Input: dimensioned drawing with shaded views. Units: mm. Origin: part minimum x, y, z. A direction names the side the tool comes from. Give positions to 0.01 mm unless a question says otherwise; leave off trailing zeros. Loops run counter-clockwise (first coordinate to the right, second up) from the corner with the lowest first, then second, coordinate; pieces in that order, holes last. Notation, with made-up numbers: (47, 2) -> (63, 2) arc R11 ccw to (63, 9) -> close; hole circle Ø3 at (77.5, 79.5). An arc over 180 degrees is marked (long way). Answer as a JSON object with one key per item and string values.
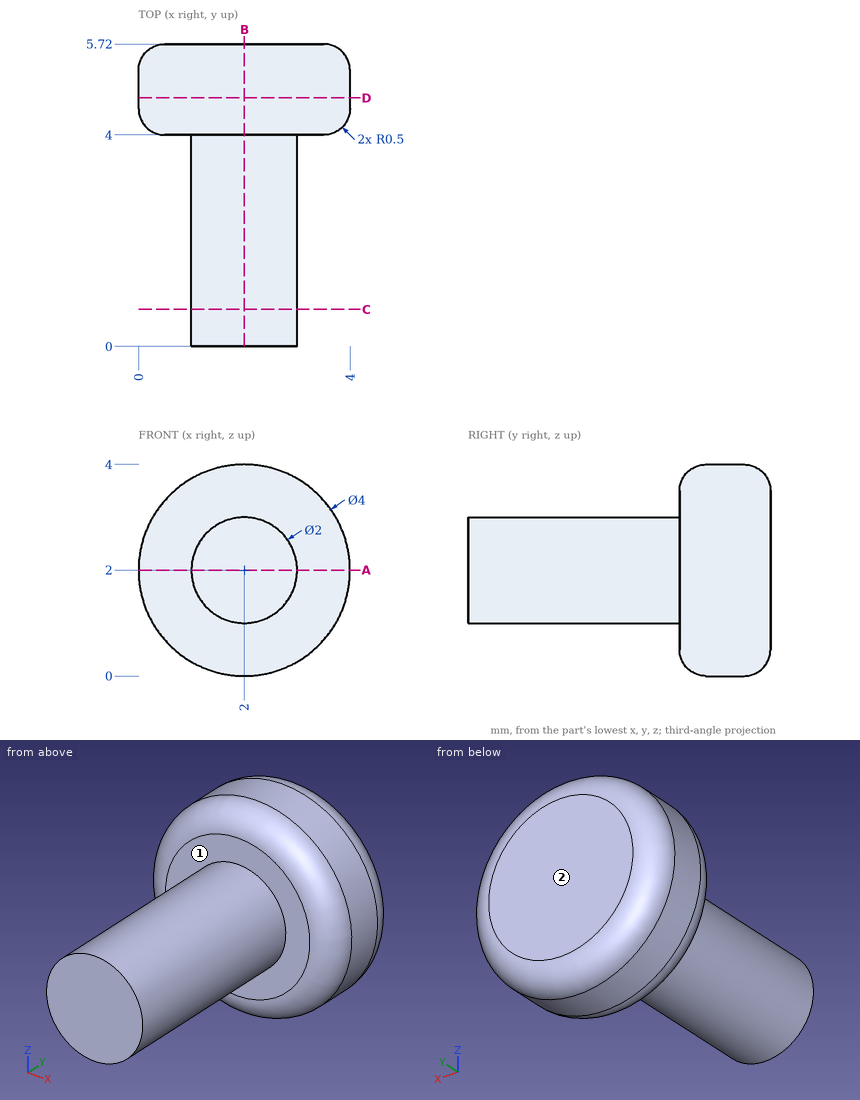
Q1. Section D-D, the plane y = 4.7. Return the cut outline in (x, z).
Evaluation:
{"outline": "circle Ø4 at (2, 2)"}
Q2. Ray query, line 1 along Y through (x, z) = (0.9, 1.8); line 2 along Z through (x, y) = (1.2, 2.3); line 3 along X through (y, z) = (4.9, 2.75). Return the intervals inside material, ascending.
Evaluation:
{"line 1": "y = 4 to 5.72", "line 2": "z = 1.4 to 2.6", "line 3": "x = 0.15 to 3.85"}
Q3. Section C-C, the plane y = 0.7. Return the cut outline in (x, z), then the cut area to 3 significant figures.
Evaluation:
{"outline": "circle Ø2 at (2, 2)", "area": "3.14 mm2"}
Q4. Section A-A, the plane z = 2. Return the cut outline in (x, y).
Evaluation:
{"outline": "(0, 4.5) arc R0.5 ccw to (0.5, 4) -> (1, 4) -> (1, 0) -> (3, 0) -> (3, 4) -> (3.5, 4) arc R0.5 ccw to (4, 4.5) -> (4, 5.22) arc R0.5 ccw to (3.5, 5.72) -> (0.5, 5.72) arc R0.5 ccw to (0, 5.22) -> close"}
Q5. Access query for the marked faces 1 and 2. Directions: +Z, -Z, +X, -X, +Y, -Y. A direction counts if a zero-diameter tool reaches every point of the face in a straight line with its end or side. Return the directions, or none.
Evaluation:
{"face 1": "-Y", "face 2": "+Z, -Z, +X, -X, +Y"}
Q6. Section B-B, the plane x = 2. Return the cut outline in (y, z).
Evaluation:
{"outline": "(0, 1) -> (4, 1) -> (4, 0.5) arc R0.5 ccw to (4.5, 0) -> (5.22, 0) arc R0.5 ccw to (5.72, 0.5) -> (5.72, 3.5) arc R0.5 ccw to (5.22, 4) -> (4.5, 4) arc R0.5 ccw to (4, 3.5) -> (4, 3) -> (0, 3) -> close"}
